Check sheet for the drawn part. Datum: minimum x, y, z corner. Units: mm. A direction names the side the tool comes from. Round coordinates to 2 decimals unless told otherwise and drop trailing zeros. Loops run counter-clockwise (first coordinate to the right, second up) from the corner with the lowest first, then second, coordinate; pieces in that order, holes last.
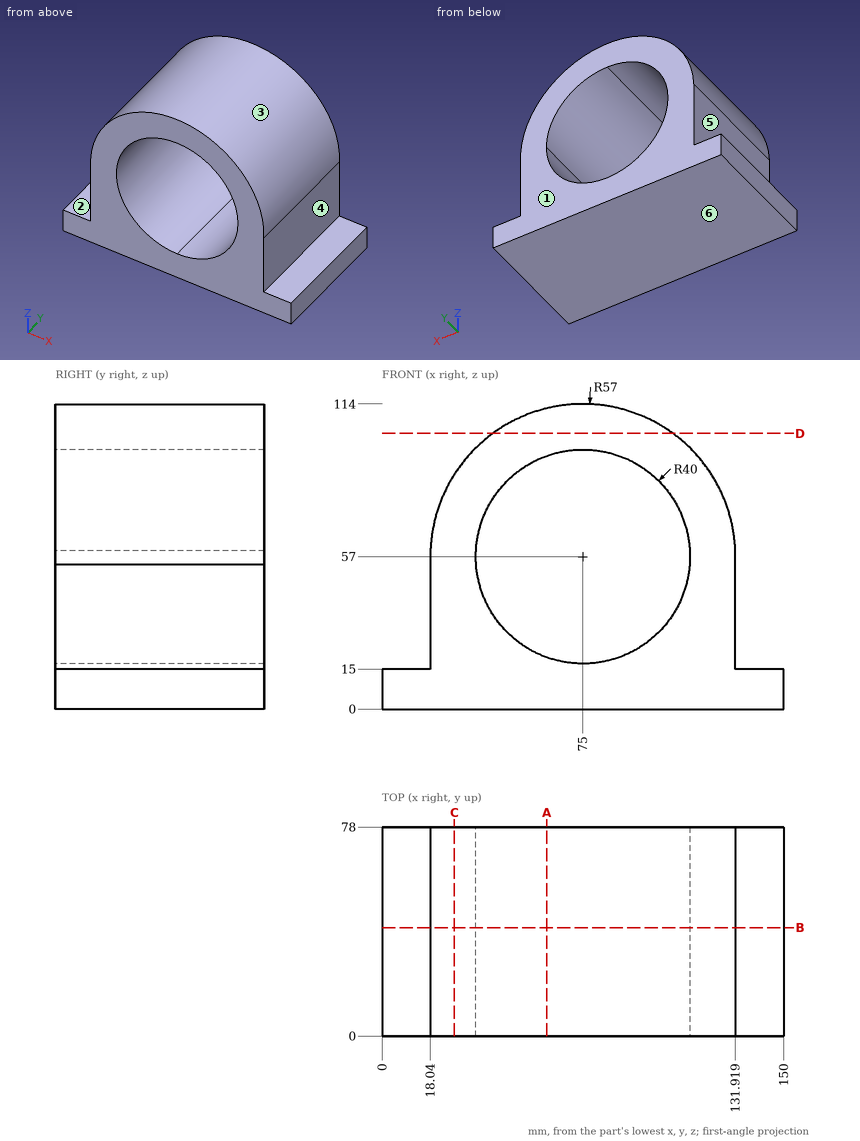
1) Sectioned sample at B-B, the plane y = 40.5. Record the cut outline in (x, z).
Report:
outline: (0, 0) - (150, 0) - (150, 15) - (131.92, 15) - (131.92, 53.96) arc R57 ccw (long way) to (18.04, 59.13) - (18.04, 15) - (0, 15) - close; hole (75, 17) arc R40 ccw to (115, 57) arc R40 ccw (long way) to start
2) Access from +Z, -Z, +X, -X, +Y, -Y to the whole of each face (thin tool, end or side, straight path). Record for the marked faces 1 and 2.
Report:
face 1: +Z, -Z, +X, -X, +Y
face 2: +Z, -X, +Y, -Y
3) Sectioned sample at D-D, the plane z = 103. Record the cut outline in (x, y), then the cut area to 3 significant figures.
Report:
outline: (41.34, 0) - (108.66, 0) - (108.66, 78) - (41.34, 78) - close
area: 5,250 mm2
4) Mould release check, pull along X, two halves, no side actions. Record for the marked faces 3, 4, 5 and 6: +X half, -X half, draft (parallel to the pull), parting line (faces both ways), or undercut.
Report:
face 3: parting line
face 4: +X half
face 5: -X half
face 6: draft
5) Sectioned sample at C-C, the plane x = 27. Record the cut outline in (y, z), then the cut area to 3 significant figures.
Report:
outline: (0, 0) - (78, 0) - (78, 87.74) - (0, 87.74) - close
area: 6,840 mm2
6) Sectioned sample at A-A, the plane x = 61.5. Record the cut outline in (y, z).
Report:
outline: (0, 0) - (78, 0) - (78, 19.35) - (0, 19.35) - close; (0, 94.65) - (78, 94.65) - (78, 112.38) - (0, 112.38) - close
7) Gauge pin test, flat ends, axial feed: pin 1 (5.5 mm diameter, centred on x = 144, y = 31, fed in from +Z); pin 2 (3 mm diameter, centred on x = 37, y = 49.5, fed in from +Z); pin 3 (8 mm diameter, centred on y = 36, z = 54, fed in from -X). Record the tip position at first contact, or that the pin passes through.
Report:
pin 1: stops at z = 15
pin 2: stops at z = 100.78
pin 3: stops at x = 18.04
8) Scan lines: line 1 along X through (y, z) = (3.5, 57.5); line 2 along Z through (x, y) = (63, 19); line 3 along X through (y, z) = (70.5, 91.5) (1 decimal). Record each from-to range of solid material in increasing order.
Report:
line 1: x = 18.04 to 35, 115 to 132
line 2: z = 0 to 18.84, 95.16 to 112.72
line 3: x = 29.6 to 54.8, 95.2 to 120.4
